from build123d import *

# Parameters (mm, degrees)
BASE_FLANGE1_DEPTH = 6.35
SKETCH8_R          = 3.4
CUT_EXTRUDE1_DEPTH = 183.851914127
SKETCH9_R          = 34
CUT_EXTRUDE2_DEPTH = 183.851914127
SKETCH10_R         = 2.75
CUT_EXTRUDE3_DEPTH = 183.851914127
TABS_1_START       = -6.35
TABS_1_DEPTH       = 6.35
TABS_2_AT_2_COUNT  = 2
TABS_2_AT_2_PITCH  = 12
CIRPATTERN2_COUNT  = 2
CIRPATTERN2_ANGLE  = 60


# Sheet-metal steps are written as plain solids
with BuildPart() as part:
    # Sketch2 → Base-Flange1 (new body)
    with BuildSketch(Plane(origin=(0, 0, 0), x_dir=(1, 0, 0), z_dir=(0, 1, 0))):
        with BuildLine():
            Line((0, 0), (50.76093065, 0))
            Line((50.76093065, 0), (107.880465325, 57.119534675))
            ThreePointArc((107.880465325, 57.119534675), (111.537953618, 118.761570635), (50.76093065, 129.682710556))
            Line((50.76093065, 129.682710556), (0, 90))
            Line((0, 90), (0, 0))
        make_face()
    extrude(amount=-BASE_FLANGE1_DEPTH)

    # Sketch8 → Cut-Extrude1 (cut, through all)
    with BuildSketch(Plane(origin=(0, 0, 0), x_dir=(1, 0, 0), z_dir=(0, 1, 0))):
        with Locations(Location((12.5, 79, 0), (0, 0, 270))):
            Circle(SKETCH8_R)
        with Locations(Location((12.5, 11, 0), (0, 0, 90))):
            Circle(SKETCH8_R)
    extrude(amount=-CUT_EXTRUDE1_DEPTH, mode=Mode.SUBTRACT)

    # Sketch9 → Cut-Extrude2 (cut, through all)
    with BuildSketch(Plane(origin=(0, 0, 0), x_dir=(1, 0, 0), z_dir=(0, 1, 0))):
        with Locations(Location((75, 90, 0), (0, 0, 270))):
            Circle(SKETCH9_R)
    extrude(amount=-CUT_EXTRUDE2_DEPTH, mode=Mode.SUBTRACT)

    # Sketch10 → Cut-Extrude3 (cut, through all)
    with BuildSketch(Plane(origin=(0, 0, 0), x_dir=(1, 0, 0), z_dir=(0, 1, 0))):
        with Locations(Location((75, 131, 0), (0, 0, 270))):
            Circle(SKETCH10_R)
        with Locations(Location((103.991378029, 118.991378029, 0), (0, 0, 270))):
            Circle(SKETCH10_R)
        with Locations(Location((116, 90, 0), (0, 0, 270))):
            Circle(SKETCH10_R)
        with Locations(Location((103.991378029, 61.008621971, 0), (0, 0, 270))):
            Circle(SKETCH10_R)
        with Locations(Location((75, 49, 0), (0, 0, 270))):
            Circle(SKETCH10_R)
        with Locations(Location((46.008621971, 61.008621971, 0), (0, 0, 270))):
            Circle(SKETCH10_R)
        with Locations(Location((34, 90, 0), (0, 0, 270))):
            Circle(SKETCH10_R)
        with Locations(Location((46.008621971, 118.991378029, 0), (0, 0, 270))):
            Circle(SKETCH10_R)
    extrude(amount=-CUT_EXTRUDE3_DEPTH, mode=Mode.SUBTRACT)

    # Sketch11 → Tabs_1 (add)
    with BuildSketch(Plane.XZ.offset(6.35).offset(TABS_1_START)):
        with BuildLine():
            Line((129, -100), (129, -80))
            ThreePointArc((129, -80), (122.450687881, -77.994187792), (118.147884423, -72.66477373))
            ThreePointArc((118.147884423, -72.66477373), (121.5, -90), (118.147884423, -107.33522627))
            ThreePointArc((118.147884423, -107.33522627), (122.450687881, -102.005812208), (129, -100))
        make_face()
    tabs_1 = extrude(amount=TABS_1_DEPTH)

    # Sketch20 → Tabs_2 (revolve, cut)
    with BuildSketch(Plane(origin=(129, -3.175, -84), x_dir=(0, 0, -1), z_dir=(0, 1, 0))):
        Polygon((0, 0), (0, 5.751075774), (1.25, 5), (1.25, 0), align=None)
    tabs_2 = revolve(axis=Axis((135.35, -3.175, -84), (-1, 0, 0)), mode=Mode.SUBTRACT)

    # Tabs_2 at 2: Tabs_2 ×2
    with Locations(*[(0, 0, -i * TABS_2_AT_2_PITCH) for i in range(1, TABS_2_AT_2_COUNT)]):
        add(tabs_2, mode=Mode.SUBTRACT)

    # CirPattern2: Tabs_1, Tabs_2 ×2 about axis
    cirpattern2_axis = Axis((75, 0, -90), (0, 1, 0))
    add([tabs_1.rotate(cirpattern2_axis, i * CIRPATTERN2_ANGLE / (CIRPATTERN2_COUNT - 1)) for i in range(1, CIRPATTERN2_COUNT)])
    add([tabs_2.rotate(cirpattern2_axis, i * CIRPATTERN2_ANGLE / (CIRPATTERN2_COUNT - 1)) for i in range(1, CIRPATTERN2_COUNT)], mode=Mode.SUBTRACT)

    # CirPattern2 copy 1 sketch → CirPattern2 copy 1 (revolve, cut)
    with BuildSketch(Plane(origin=(96.803847577, -3.175, -139.765371804), x_dir=(-0.8660254037844399, 0, -0.4999999999999978), z_dir=(0, 1, 0))):
        Polygon((0, 0), (0, 5.751075774), (1.25, 5), (1.25, 0), align=None)
    revolve(axis=Axis((99.978847577, -3.175, -145.264633118), (-0.4999999999999978, 0, 0.8660254037844399)), mode=Mode.SUBTRACT)


solid = part.part
Geometry check sheet. Reference: the model listing, model coordinates, mm. Round coordinates to 2 decimals unless told otherwise and drop trailing zeros. Loops run counter-clockwise (first coordinate to the right, second up) from the corner with the lowest first, then second, coordinate; pieces in that order, holes last. Notation, with made-up numbers: (47.5, -8.5) -> (53.5, -8.5) arc R19 ccw to (53.5, 20.5) -> close; hole circle Ø3 at (19.25, 10.25). An arc over 180 degrees is marked (long way). Answer as a JSON object with one key per item and string values. Group by question number.
Item 1: Release check for a two-part mould opening along Z. For faces 1 (the face through (25, -3, 0)), 2 (the face through (104.11, -3.13, -121.74)), 3 (the face through (122.37, -3.13, -102.06)) record: pulls with the +Z half, pulls with the -Z half, needs draft (parallel to the pull), parting line crosses it, or undercut.
Item 2: Thickness scan on line 1 along X through (y, z) = (-2, -90); line 2 along X through (y, z) = (-5.5, -81); line 3 along Z through (x, y) = (48.5, -3.75). Record the ranges inside material, lowest first.
Item 3: Depth check by flat-ended pin: pin 1 Ø1.5 at (x, y) = (72.5, -4) entering from +Z; pin 2 Ø2 at (y, z) = (-3.175, -84) entering from +X; pin 3 Ø3.5 at (x, z) = (75, -49) entering from -Y; pin 4 Ø1.5 at (x, y) = (21.5, -1.5) entering from -Z. Enter the tip coordinate at first touch or a pass-through.
Item 4: Cross-section at C-C, the plane x = 12.5. Record the cut outline in (y, z).
Item 5: Cross-section at B-B, the plane z = -69.5. Record the cut outline in (x, y), plus the area to 3 significant figures.
Item 6: Cross-section at D-D, the plane x = 55. Record the cut outline in (y, z), plus the area to 3 significant figures.
Item 7: Cross-section at A-A, the plane x = 75. Record the cut outline in (y, z).
Determined:
{
 "1": {"face 1": "pulls with the +Z half", "face 2": "undercut", "face 3": "pulls with the -Z half"},
 "2": {"line 1": "x = 0 to 31.25, 36.75 to 41, 109 to 113.25, 118.75 to 129", "line 2": "x = 0 to 9.75, 15.25 to 42.21, 107.79 to 129", "line 3": "z = -127.92 to -120.16, -117.83 to -111.3, -68.7 to -62.17, -59.84 to 0"},
 "3": {"pin 1": "stops at z = -20.99", "pin 2": "stops at x = 123.85", "pin 3": "passes through", "pin 4": "stops at z = -107.39"},
 "4": {"outline": "(-6.35, -99.77) -> (0, -99.77) -> (0, -82.4) -> (-6.35, -82.4) -> close; (-6.35, -75.6) -> (0, -75.6) -> (0, -14.4) -> (-6.35, -14.4) -> close; (-6.35, -7.6) -> (0, -7.6) -> (0, 0) -> (-6.35, 0) -> close"},
 "5": {"outline": "(0, -6.35) -> (47.88, -6.35) -> (47.88, 0) -> (0, 0) -> close; (102.12, -6.35) -> (116.74, -6.35) -> (116.74, 0) -> (102.12, 0) -> close", "area": "397 mm²"},
 "6": {"outline": "(-6.35, -131.98) -> (0, -131.98) -> (0, -117.5) -> (-6.35, -117.5) -> close; (-6.35, -62.5) -> (0, -62.5) -> (0, -4.24) -> (-6.35, -4.24) -> close", "area": "462 mm²"},
 "7": {"outline": "(-6.35, -136.5) -> (0, -136.5) -> (0, -133.75) -> (-6.35, -133.75) -> close; (-6.35, -128.25) -> (0, -128.25) -> (0, -124) -> (-6.35, -124) -> close; (-6.35, -56) -> (0, -56) -> (0, -51.75) -> (-6.35, -51.75) -> close; (-6.35, -46.25) -> (0, -46.25) -> (0, -24.24) -> (-6.35, -24.24) -> close"}
}
